from build123d import *

# Parameters (mm, degrees)
BOSS_EXTRUDE1_DEPTH = 55
SKETCH2_W           = 4
SKETCH2_H           = 55
SKETCH6_R           = 2.5
CUT_EXTRUDE1_DEPTH  = 10
SKETCH7_W           = 10
SKETCH7_H           = 31.5
CUT_EXTRUDE2_DEPTH  = 10
SKETCH8_W           = 9.818662261
SKETCH8_H           = 11
CUT_EXTRUDE3_DEPTH  = 69.208914829
BOSS_EXTRUDE2_START = -3.6
SKETCH9_R           = 2.8
SKETCH9_R_2         = 1.7
BOSS_EXTRUDE2_DEPTH = 7


with BuildPart() as part:
    # Sketch1 → Boss-Extrude1 (new body)
    with BuildSketch(Plane(origin=(0, 0, 0), x_dir=(1, 0, 0), z_dir=(0, 1, 0))):
        Polygon((-4.182050808, 7.243524479), (-8.364101615, 0), (-4.182050808, -7.243524479), (4.182050808, -7.243524479), (8.364101615, 0), (4.182050808, 7.243524479), align=None)
        Polygon((-4.9, 0), (-2.45, -4.243524479), (2.45, -4.243524479), (4.9, 0), (2.45, 4.243524479), (-2.45, 4.243524479), align=None, mode=Mode.SUBTRACT)
    extrude(amount=BOSS_EXTRUDE1_DEPTH)

    # Sweep1: sweep along a path in Sketch3
    with BuildLine(Plane(origin=(0, 55, 0), x_dir=(1, 0, 0), z_dir=(0, 1, 0))) as sweep1_path:
        Line((6.273076211, 3.621762239), (7.139101615, 4.121762239))
        ThreePointArc((7.139101615, 4.121762239), (13.761110972, 12.313986191), (13.182050808, 22.831981747))
        ThreePointArc((13.182050808, 22.831981747), (10.196814467, 27.168510904), (5.872312911, 30.17114432))
    # Sketch2 → Sweep1 (sweep)
    with BuildSketch(Plane(origin=(6.273076211, 0, -3.621762239), x_dir=(-0.5000000000000001, 0, -0.8660254037844386), z_dir=(0.8660254037844386, 0, -0.5000000000000001))):
        with Locations((0, 27.5)):
            Rectangle(SKETCH2_W, SKETCH2_H)
    sweep(path=sweep1_path.line)

    # Sketch6 → Cut-Extrude1 (cut)
    with BuildSketch(Plane(origin=(17.267694528, 0, -0.839732793), x_dir=(-0.0485728772715999, 0, -0.9988196411732992), z_dir=(0.9988196411732992, 0, -0.0485728772715999))):
        with Locations((16.810213392, 46.05)):
            Circle(SKETCH6_R)
        with Locations((16.810213392, 8.95)):
            Circle(SKETCH6_R)
    extrude(amount=-CUT_EXTRUDE1_DEPTH, mode=Mode.SUBTRACT)

    # Sketch7 → Cut-Extrude2 (cut)
    with BuildSketch(Plane(origin=(17.267694528, 0, -0.839732793), x_dir=(-0.0485728772715999, 0, -0.9988196411732992), z_dir=(0.9988196411732992, 0, -0.0485728772715999))):
        with Locations((16.810213392, 27.5)):
            Rectangle(SKETCH7_W, SKETCH7_H)
    extrude(amount=-CUT_EXTRUDE2_DEPTH, mode=Mode.SUBTRACT)

    # Sketch8 → Cut-Extrude3 (cut, through all)
    with BuildSketch(Plane(origin=(17.267694528, 0, -0.839732793), x_dir=(-0.0485728772715999, 0, -0.9988196411732992), z_dir=(0.9988196411732992, 0, -0.0485728772715999))):
        with Locations((26.719544523, 27.5)):
            Rectangle(SKETCH8_W, SKETCH8_H)
    extrude(amount=-CUT_EXTRUDE3_DEPTH, mode=Mode.SUBTRACT)

    # Sketch9 → Boss-Extrude2 (add)
    # profile 1 of 2: a face of its own
    with BuildSketch(Plane(origin=(17.267694528, 0, -0.839732793), x_dir=(-0.0485728772715999, 0, -0.9988196411732992), z_dir=(0.9988196411732992, 0, -0.0485728772715999)).offset(BOSS_EXTRUDE2_START)):
        with Locations((16.810213392, 46.05)):
            Circle(SKETCH9_R)
        with Locations(Location((16.810213392, 46.05, 0), (0, 0, 180))):
            Circle(SKETCH9_R_2, mode=Mode.SUBTRACT)
    # profile 2 of 2: a face of its own
    with BuildSketch(Plane(origin=(17.267694528, 0, -0.839732793), x_dir=(-0.0485728772715999, 0, -0.9988196411732992), z_dir=(0.9988196411732992, 0, -0.0485728772715999)).offset(BOSS_EXTRUDE2_START)):
        with Locations(Location((16.810213392, 8.95, 0), (0, 0, 90.000000002))):
            Circle(SKETCH9_R)
        with Locations((16.810213392, 8.95)):
            Circle(SKETCH9_R_2, mode=Mode.SUBTRACT)
    extrude(amount=-BOSS_EXTRUDE2_DEPTH)


solid = part.part
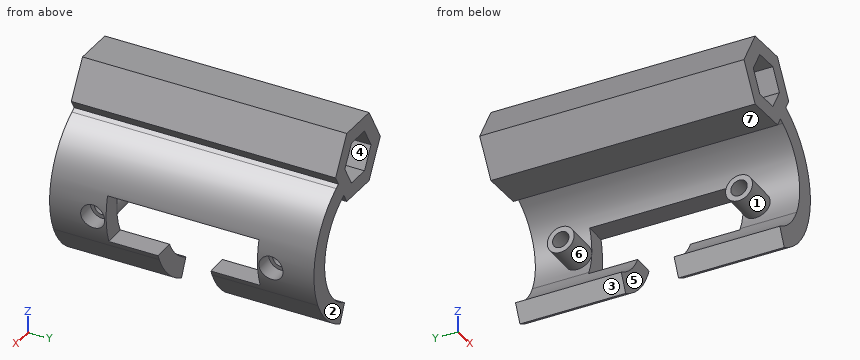
Design review of the part built by this model. Coordinates are the model's own, in mm. Face numbers are marked on the shaded views. A direction names the side the tool comes from. Round coordinates to 2 decimals unless told otherwise and drop trailing zeros. Order: outer loops, then holes, each group sorted by start corner. A loop starts at its lowest first (then second) coordinate and runs counter-clockwise, first axis right, second up.
1) Consider section A-A (y = 15.5). State the section outline as (x, z) points, plus the area to 3 significant figures.
The answers:
outline: (-8.36, 0) - (-4.18, -7.24) - (4.18, -7.24) - (5.27, -5.35) - (6.14, -5.85) arc R12.66 cw to (11.67, -12.39) - (15.93, -12.6) arc R16.66 ccw to (8.14, -2.39) - (7.27, -1.89) - (8.36, 0) - (4.18, 7.24) - (-4.18, 7.24) - close; (5.05, -28.35) - (6.7, -31.99) arc R16.66 ccw to (15.44, -22.59) - (11.19, -22.38) arc R12.66 cw to start; hole (-4.9, 0) - (-2.45, -4.24) - (2.45, -4.24) - (4.9, 0) - (2.45, 4.24) - (-2.45, 4.24) - close
area: 211 mm2
2) Consider section D-D (y = 4). State the section outline as (x, z) points.
The answers:
outline: (-8.36, 0) - (-4.18, -7.24) - (4.18, -7.24) - (5.27, -5.35) - (6.14, -5.85) arc R12.66 cw to (5.05, -28.35) - (6.7, -31.99) arc R16.66 ccw to (8.14, -2.39) - (7.27, -1.89) - (8.36, 0) - (4.18, 7.24) - (-4.18, 7.24) - close; hole (-4.9, 0) - (-2.45, -4.24) - (2.45, -4.24) - (4.9, 0) - (2.45, 4.24) - (-2.45, 4.24) - close
3) Consider section C-C (z = -27). State the section outline as (x, y) points, plus the area to 3 significant figures.
The answers:
outline: (7.34, 0) - (13, 0) - (13, 22) - (7.34, 22) - close; (7.34, 33) - (13, 33) - (13, 55) - (7.34, 55) - close
area: 249 mm2
4) Clearance check with flat-ended pins moving along their axes: pin 1 Ø5.5 at (x, y) = (1, 37.5) entering from -Z; pin 2 Ø2 at (x, y) = (8.5, 38) entering from +Z; pin 3 Ø1 at (x, y) = (6, 17) entering from -Z; pin 4 Ø10 at (x, z) = (-3, 1.5) entering from +Y. State where each tip first meets the part, or that it passes through.
The answers:
pin 1: stops at z = -7.24
pin 2: stops at z = 1.5
pin 3: stops at z = -31.55
pin 4: stops at y = 55
5) Machinability: for the marked faces 4, 5, 6 and 7, which of the approach directions +Z, -Z, +X, -X, +Y, -Y give a long, thin tool a straight path to every point of the face, cutting with its end or side? Answer none if there is none.
The answers:
face 4: +Y, -Y
face 5: -Z, +X, -X
face 6: none
face 7: -Z, -X, +Y, -Y
6) Consider section B-B (x = 1.25). State the section outline as (y, z) points, plus the area to 3 significant figures.
The answers:
outline: (0, -7.24) - (55, -7.24) - (55, -4.24) - (0, -4.24) - close; (0, 4.24) - (55, 4.24) - (55, 7.24) - (0, 7.24) - close
area: 330 mm2
7) Draft analysis for pull direction Y (two halves, no side actions). For the marked faces 1, 2 and 3, state which applies: released by +Y, released by -Y, zero draft, split by the parting line, or undercut.
The answers:
face 1: undercut
face 2: released by +Y
face 3: zero draft
8) For L1, parallel to Y at x = 10, z = -28; L2, parallel to Z at x = -0.75, y = 42.5; L3, parallel to X at y = 30, z = -1.5, list the stretches that pass through material, from the lowest coordinate up.
The answers:
L1: y = 0 to 22, 33 to 55
L2: z = -7.24 to -4.24, 4.24 to 7.24
L3: x = -7.5 to -4.03, 4.03 to 7.5
